Work out the finished part from the listing and answer in its coordinate system (mm). A direction names the side the tool comes from. Round coordinates to 2 decimals unless told otherwise and drop trailing zeros. Loops run counter-clockwise (first coordinate to the right, second up) from the corner with the lowest first, then second, coordinate; pieces in that order, holes last. Notation, with made-up numbers: (28.5, 27) - (80.5, 27) arc R11 cw to (80.5, 34) - close; hole circle Ø6 at (71, -14). An arc over 180 degrees is marked (long way). Answer as CSV lines item,"result". Start each with the question number.
Q1. Each of these flat-tipped pins is pushed along its axis until it touches: pin 1 Ø1.7 at (x, z) = (17.5, -45.5) entering from -Y; pin 2 Ø4 at (x, z) = (19, -46.5) entering from -Y; pin 3 Ø2 at (y, z) = (-20, -43.5) entering from -X (3 decimals). Where does it stop, or does it pass through?
Q2. For faces 1 (the face through (-9.99, -10.23, -45.07)), 2 (the face through (-16.5, -21.375, -47.3)), 3 (the face through (20, -19.375, -46)), determine the directions among +Z, -Z, +X, -X, +Y, -Y from which every point of the face is accessible in a straight line to the end or side of a thin tool.
Q3. Section A-A on x = 18.5 is taken. Write down the section's boundary in (y, z).
Q4. The mould has two halves that part along Z. Classify faces 4 (the face through (-18.825, -15.608, -46.464)), 5 (the face through (0.1, -23.3, -40)), 6 (the face through (20.5, -21.375, -47.3)), 7 (the face through (0.1, -23.3, -50)): +Z half, -Z half, draft (parallel to the pull), parting line (faces both ways), or undercut.
Q5. Section B-B on y = -10.25 is taken. Write down the section's boundary in (x, z), then the cut area to 3 significant figures.
Q6. Straight lines are drawn through the part: L1, parallel to Z at x = -18.5, y = -16; L2, parallel to X at y = -13.5, z = -45; L3, parallel to X at y = -20.5, z = -43 (3 decimals). For each, find the intervals that lie inside material, in ascending order. Write a range as [from, to].
Q7. Section C-C on z = -45 is taken. Count the separate pieces of the cut face and the enclosed holes in it, then the cut area to 3 significant figures.
```python
from build123d import *

# Parameters (mm, degrees)
PAD017_DEPTH         = 10
SKETCH027_R          = 1.5
POCKET015_DEPTH      = 0.001
POCKET015_DEPTH_BACK = 26.046246
SKETCH028_R          = 2.85
POCKET016_DEPTH      = 2


with BuildPart() as part:
    # Sketch026 → Pad017 (new body)
    with BuildSketch(Plane.XY):
        with BuildLine():
            ThreePointArc((-21.365, -18.875435), (-25.083946, -13.547727), (-27.5, -7.516333))
            ThreePointArc((-27.5, -7.516333), (-19.604248, -11.995431), (-10.983083, -9.152768))
            ThreePointArc((-10.983083, -9.152768), (-9.977451, -10.239713), (-8.864785, -11.216811))
            add(Edge.make_bspline(
                [(8.864785, -11.216811), (0, -35.083189), (-8.864785, -11.216811)],
                knots=[-8.864785, -8.864785, -8.864785, 8.864785, 8.864785, 8.864785], degree=2))
            ThreePointArc((8.864785, -11.216811), (9.977451, -10.239713), (10.983083, -9.152768))
            ThreePointArc((10.983083, -9.152768), (19.604248, -11.995431), (27.5, -7.516333))
            ThreePointArc((27.5, -7.516333), (25.083946, -13.547727), (21.365, -18.875435))
            Line((21.365, -18.875435), (21.365, -21.375435))
            Line((21.365, -21.375435), (15.635, -21.375435))
            ThreePointArc((15.635, -21.375435), (0, -26.045246), (-15.635, -21.375435))
            Line((-15.635, -21.375435), (-21.365, -21.375435))
            Line((-21.365, -21.375435), (-21.365, -18.875435))
        make_face()
    extrude(amount=PAD017_DEPTH)

    # Sketch027 → Pocket015 (cut, two sides)
    with BuildSketch(Plane.XZ) as pocket015_sk:
        with Locations((-18.5, 5)):
            Circle(SKETCH027_R)
        with Locations((18.5, 5)):
            Circle(SKETCH027_R)
    extrude(amount=-POCKET015_DEPTH, mode=Mode.SUBTRACT)
    extrude(pocket015_sk.sketch, amount=POCKET015_DEPTH_BACK, mode=Mode.SUBTRACT)

    # Sketch028 (on DatumPlane) → Pocket016 (cut)
    with BuildSketch(Plane.XZ.offset(21.375435)):
        with Locations((-18.5, 5)):
            Circle(SKETCH028_R)
        with Locations((18.5, 5)):
            Circle(SKETCH028_R)
    extrude(amount=-POCKET016_DEPTH, mode=Mode.SUBTRACT)


with BuildPart() as part_1:
    # Body008 placement: moved
    add(part.part.moved(Location((0, 0, -50))))


solid = part_1.part
```
Findings:
1,pin 1,"stops at y = -19.38"
1,pin 2,"stops at y = -21.38"
1,pin 3,"stops at x = -21.365"
2,face 1,"+Z, -Z, +Y"
2,face 2,"+Z, -Z, -X, -Y"
2,face 3,"-Y"
3,outline,"(-21.38, -50) - (-12.05, -50) - (-12.05, -46.5) - (-19.38, -46.5) - (-19.38, -47.85) - (-21.38, -47.85) - close; (-21.38, -42.15) - (-19.38, -42.15) - (-19.38, -43.5) - (-12.05, -43.5) - (-12.05, -40) - (-21.38, -40) - close"
4,face 4,"undercut"
4,face 5,"+Z half"
4,face 6,"draft"
4,face 7,"-Z half"
5,outline,"(-26.6, -50) - (-24.59, -50) - (-24.59, -40) - (-26.6, -40) - close; (-12.41, -50) - (-9.97, -50) - (-9.97, -40) - (-12.41, -40) - close; (9.97, -50) - (12.41, -50) - (12.41, -40) - (9.97, -40) - close; (24.59, -50) - (26.6, -50) - (26.6, -40) - (24.59, -40) - close"
5,area,"89.1 mm^2"
6,L1,"z = [-50, -46.5], [-43.5, -40]"
6,L2,"x = [-25.11, -20], [-17, -7.97], [7.97, 17], [20, 25.11]"
6,L3,"x = [-21.365, -20.53], [-16.47, -4.177], [4.177, 16.47], [20.53, 21.365]"
7,separate pieces,"3"
7,enclosed holes,"0"
7,area,"377 mm^2"
